Geometry check sheet. Reference: drawing and pictorial views, mm from the part's lowest x, y, z. A direction names the side the tool comes from. Give positions to 0.01 mm unless a question says otherwise; leave off trailing zeros. Write each loop counter-clockwise with the first axis right and the second up, starting at its lowest first coordinate (ties: lowest second). Pieces come first, ordered by that corner, then holes. Notation, with made-up numbers: (-14.5, 41.25) - (-10.5, 41.25) arc R5 cw to (-10.5, 45.25) - close; hole circle Ø6 at (24, -10.75). An arc over 180 degrees is marked (long way). Put each result on its own line as item: value.
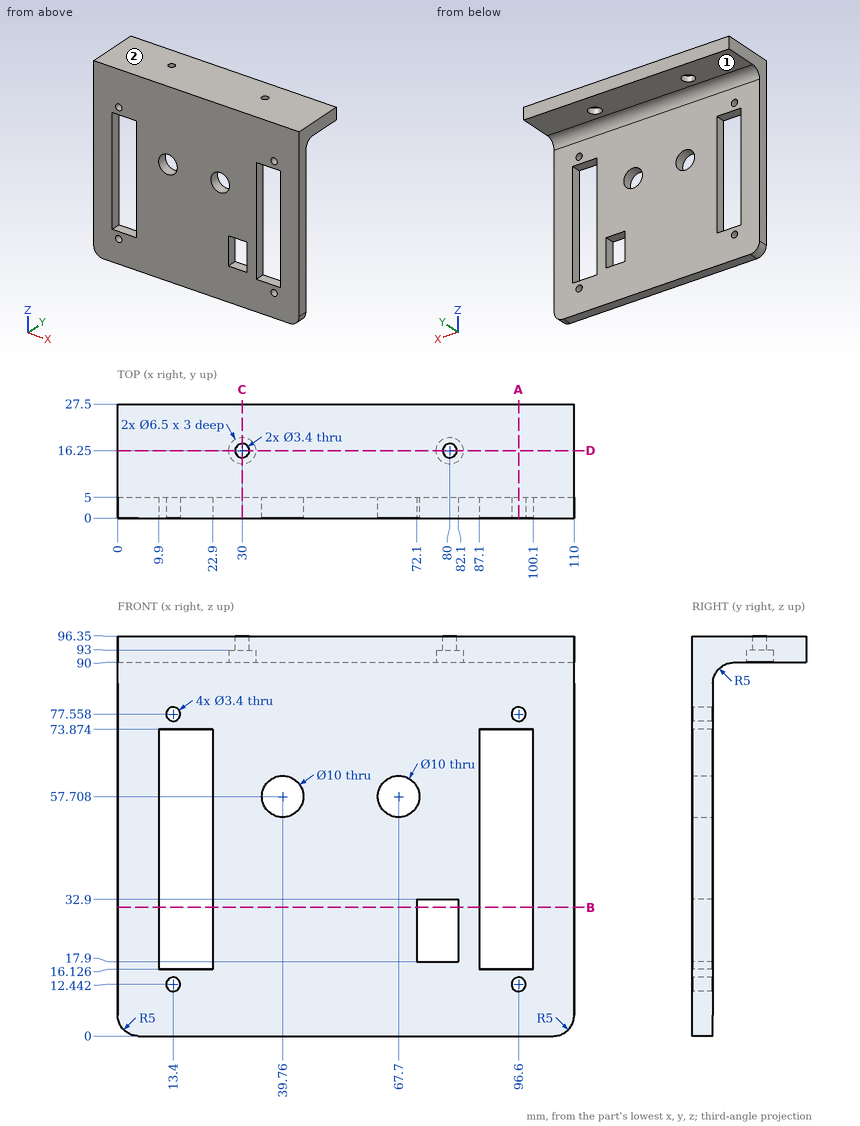
Q1. Scan lines: line 1 along Z through (x, y) = (96.6, 3.35); line 2 along Z through (x, y) = (67.7, 2); line 3 along Z through (x, y) = (88.5, 2.5). Record each from-to range of solid material in increasing order.
Answers follow:
line 1: z = 0 to 10.74, 14.14 to 16.13, 73.87 to 75.86, 79.26 to 96.35
line 2: z = 0 to 52.71, 62.71 to 96.35
line 3: z = 0 to 16.13, 73.87 to 96.35
Q2. Section check C-C, the plane x = 30. Record the cut outline in (y, z), plus the area to 3 significant figures.
Answers follow:
outline: (0, 0) - (5, 0) - (5, 85) arc R5 cw to (10, 90) - (13, 90) - (13, 93) - (14.55, 93) - (14.55, 96.35) - (0, 96.35) - close; (17.95, 93) - (19.5, 93) - (19.5, 90) - (27.5, 90) - (27.5, 96.35) - (17.95, 96.35) - close
area: 599 mm2
Q3. Go/stop test with flat-tipped pins: pin 1 Ø3 at (x, z) = (45.5, 62) entering from +Y; pin 2 Ø7 at (x, y) = (31, 15.5) entering from -Z; pin 3 Ø2 at (x, y) = (80.5, 17.5) entering from -Z. Record where each tip stops, or that it passes through.
Answers follow:
pin 1: stops at y = 5
pin 2: stops at z = 90
pin 3: stops at z = 93
Q4. Section check A-A, the plane x = 96.6. Record the cut outline in (y, z).
Answers follow:
outline: (0, 0) - (5, 0) - (5, 10.74) - (0, 10.74) - close; (0, 14.14) - (5, 14.14) - (5, 16.13) - (0, 16.13) - close; (0, 73.87) - (5, 73.87) - (5, 75.86) - (0, 75.86) - close; (0, 79.26) - (5, 79.26) - (5, 85) arc R5 cw to (10, 90) - (27.5, 90) - (27.5, 96.35) - (0, 96.35) - close
Q5. Section check B-B, the plane z = 31. Record the cut outline in (x, y), plus the area to 3 significant figures.
Answers follow:
outline: (0, 0) - (9.9, 0) - (9.9, 5) - (0, 5) - close; (22.9, 0) - (72.1, 0) - (72.1, 5) - (22.9, 5) - close; (82.1, 0) - (87.1, 0) - (87.1, 5) - (82.1, 5) - close; (100.1, 0) - (110, 0) - (110, 5) - (100.1, 5) - close
area: 370 mm2
Q6. Set-up check for the marked faces 1 and 2: record each of +Z, -Z, +X, -X, +Y, -Y from which the full face is reachable in a straight line by a thin tool's end or side.
Answers follow:
face 1: -Z, +X, -X, +Y
face 2: +Z, +X, -X, +Y, -Y
Q7. Section check D-D, the plane y = 16.25. Record the cut outline in (x, z).
Answers follow:
outline: (0, 90) - (26.75, 90) - (26.75, 93) - (28.3, 93) - (28.3, 96.35) - (0, 96.35) - close; (31.7, 93) - (33.25, 93) - (33.25, 90) - (76.75, 90) - (76.75, 93) - (78.3, 93) - (78.3, 96.35) - (31.7, 96.35) - close; (81.7, 93) - (83.25, 93) - (83.25, 90) - (110, 90) - (110, 96.35) - (81.7, 96.35) - close
